from build123d import *

# Parameters (mm, degrees)
F1_DEPTH = 50.8
F3_D     = 25.4
F4_T     = -2.54


with BuildPart() as f1:
    # F0 (on Top) → F1 (new body)
    with BuildSketch(Plane.XY):
        with BuildLine():
            Line((88.9, 38.1), (-88.9, 38.1))
            ThreePointArc((-88.9, 38.1), (-115.840768, 26.940768), (-127, 0))
            ThreePointArc((-127, 0), (-115.840768, -26.940768), (-88.9, -38.1))
            Line((-88.9, -38.1), (88.9, -38.1))
            ThreePointArc((88.9, -38.1), (115.840768, -26.940768), (127, 0))
            ThreePointArc((127, 0), (115.840768, 26.940768), (88.9, 38.1))
        make_face()
    extrude(amount=F1_DEPTH)

    # F3 (through all)
    with Locations(Plane.XY.offset(50.8)):
        with Locations((-88.9, 0), (88.9, 0)):
            Hole(F3_D / 2)

    # F4
    f4_openings = [f1.faces().sort_by_distance(p)[0] for p in [
        (0, 0, 0),
    ]]
    offset(amount=F4_T, openings=f4_openings)


solid = f1.part
Read the model definition and answer for the solid it produces. Units are mm, in the model's axes. A direction names the side the tool comes from. Give positions to 0.01 mm unless a question says otherwise; leave off trailing zeros. Write each loop counter-clockwise with the first axis right and the second up, starting at its lowest first coordinate (ties: lowest second). Pieces come first, ordered by that corner, then holes. Notation, with made-up numbers: M 66.25,-39 L 113.25,-39 A20 cw 113.25,-14 Z; hole C 8,39 d4. An arc over 180 degrees is marked long. One line per item, written item: value. Start each with the question number.
(1) Find section A-A (z = 37.5). Determine the outline of the cut face in (x, y).
(2) Determine the mould class of faces 3 (the flat face through (-1, -38.1, 25)), 4 (the flat face through (-92.4, 12.5, 0)), 5 (the flat face through (-1, -35.56, 24)), 6 (the cylindrical face through (-101.014, 3.815, 25.044)) for opening direction Y: pulls with the +Y half, pulls with the -Y half, needs draft (parallel to the pull), parting line crosses it, or undercut.
(3) Find section C-C (x = -15.5). Determine the outline of the cut face in (y, z).
(4) Find the intervals of material crossed by line 1 (Y direction, x = -88.9, z = 30.5); line 2 (X direction, y = -1, z = 16); line 3 (Y direction, x = 8.5, z = 17), in increasing order.
(5) Find section D-D (y = -23.5). Determine the outline of the cut face in (x, z).
(6) A tool of negligible diameter and unlimited length cuts with its end or side. For faces 1 (the flat face through (-1, -37, 0)), 2 (the cylindrical face through (100.994, -9.273, 23.792)), from which of +Z, -Z, +X, -X, +Y, -Y can it reach the whole face along a straight path? Write none if from no direction.
(7) Find section B-B (x = -81). Determine the outline of the cut face in (y, z).
(8) Flat-ended cylindrical pins translate along their axes: pin 1 Ø4 at (x, z) = (101.5, 20) entering from +Y; pin 2 Ø1.5 at (x, z) = (-94.5, 28) entering from -Y; pin 3 Ø21.5 at (x, y) = (6, 15) entering from -Z. Find the tip coordinate at first contact, or state that the pin passes through.
Results below:
1. outline: M -127,0 A38.1 ccw -88.9,-38.1 L 88.9,-38.1 A38.1 ccw 127,0 A38.1 ccw 88.9,38.1 L -88.9,38.1 A38.1 ccw Z; C -88.9,0 d30.48; C 88.9,0 d30.48; hole M -124.46,0 A35.56 ccw -88.9,-35.56 L 88.9,-35.56 A35.56 ccw 124.46,0 A35.56 ccw 88.9,35.56 L -88.9,35.56 A35.56 ccw Z; hole C -88.9,0 d25.4; hole C 88.9,0 d25.4
2. face 3: pulls with the -Y half
2. face 4: needs draft
2. face 5: undercut
2. face 6: undercut
3. outline: M -38.1,0 L -35.56,0 L -35.56,48.26 L 35.56,48.26 L 35.56,0 L 38.1,0 L 38.1,50.8 L -38.1,50.8 Z
4. line 1: y = -38.1 to -35.56, -15.24 to -12.7, 12.7 to 15.24, 35.56 to 38.1
4. line 2: x = -126.99 to -124.45, -104.11 to -101.56, -76.24 to -73.69, 73.69 to 76.24, 101.56 to 104.11, 124.45 to 126.99
4. line 3: y = -38.1 to -35.56, 35.56 to 38.1
5. outline: M -118.89,0 L -115.59,0 L -115.59,48.26 L 115.59,48.26 L 115.59,0 L 118.89,0 L 118.89,50.8 L -118.89,50.8 Z
6. face 1: -Z, +X, -X, +Y, -Y
6. face 2: -Z
7. outline: M -38.1,0 L -35.56,0 L -35.56,48.26 L -13.03,48.26 L -13.03,0 L -9.94,0 L -9.94,50.8 L -38.1,50.8 Z; M 9.94,0 L 13.03,0 L 13.03,48.26 L 35.56,48.26 L 35.56,0 L 38.1,0 L 38.1,50.8 L 9.94,50.8 Z
8. pin 1: stops at y = 36.6
8. pin 2: stops at y = -37.79
8. pin 3: stops at z = 48.26
